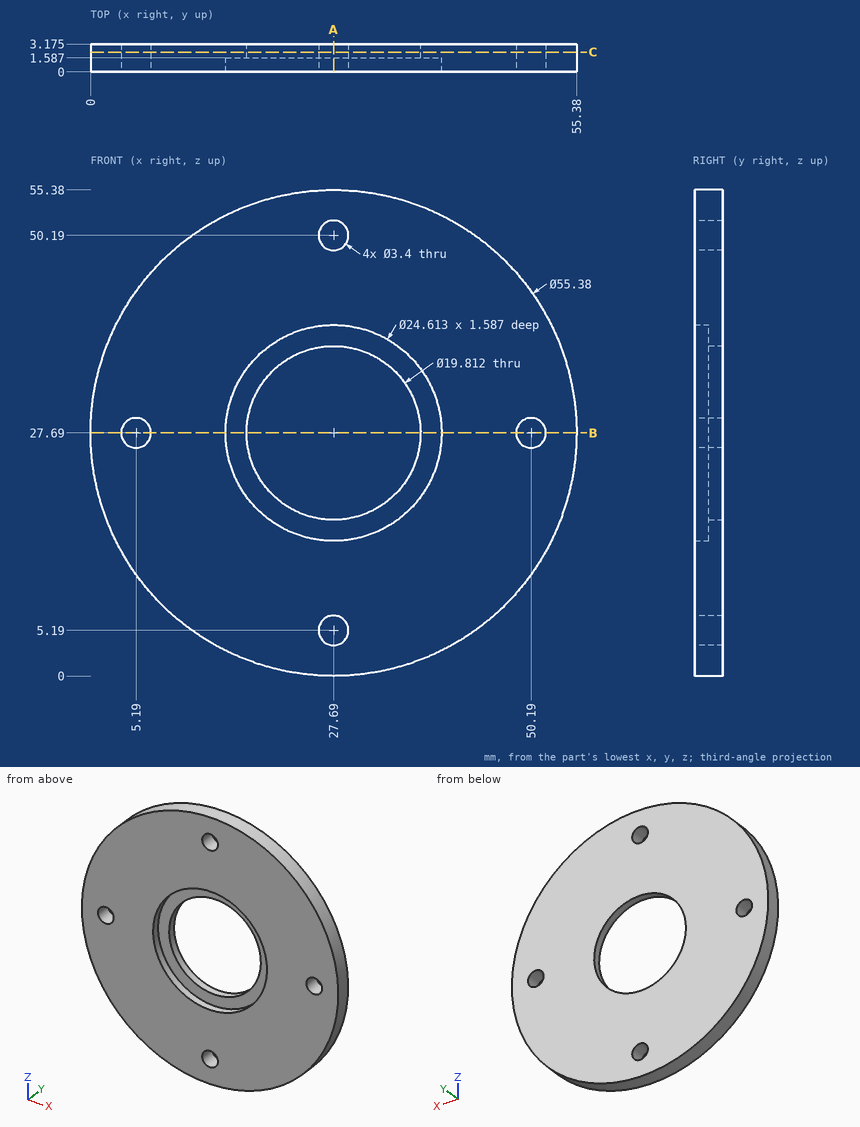
Study the drawing (mm; zero at the part's minimum x, y, z) and answer. Coordinates: 2 decimals unless noted, no trailing zeros. Loops run counter-clockwise (first coordinate to the right, second up) from the corner with the lowest first, then second, coordinate; pieces in that order, holes last. Notation, with made-up numbers: (-24.75, 14.5) -> (7.25, 14.5) arc R25 cw to (7.25, 49.5) -> close; hole circle Ø10 at (68, 65.25). An arc over 180 degrees is marked (long way). Answer in a Markdown table with one row per item. Add a question column.
1. The part is cut by section A-A, the plane x = 27.69. Write down the section's boundary in (y, z) (1 decimal).
2. A flat-ended cylindrical pin translates along its axis: P1, Ø2, axis at x = 50.19, z = 27.69, coming from the +Y side. Find the tip coordinate at first contact, or state that the pin passes through.
3. The part is cut by section C-C, the plane y = 2.25. Write down the section's boundary in (x, z) (1 decimal), then the cut area to 3 significant figures.
4. The part is cut by section B-B, the plane z = 27.69. Write down the section's boundary in (x, y) (1 decimal).
5. Consider line 1 (X direction, y = 2.6, z = 27.69) (1 decimal); line 2 (X direction, y = 1, z = 27.69); line 3 (X direction, y = 1.9, z = 4.5) (1 decimal). Determine where each line is inside the solid, lowest interval first. Write a range as [from, to].
Answer below:
| question | item | result |
|---|---|---|
| 1 | outline | (0, 0) -> (3.2, 0) -> (3.2, 3.5) -> (0, 3.5) -> close; (0, 6.9) -> (3.2, 6.9) -> (3.2, 17.8) -> (1.6, 17.8) -> (1.6, 15.4) -> (0, 15.4) -> close; (0, 40) -> (1.6, 40) -> (1.6, 37.6) -> (3.2, 37.6) -> (3.2, 48.5) -> (0, 48.5) -> close; (0, 51.9) -> (3.2, 51.9) -> (3.2, 55.4) -> (0, 55.4) -> close |
| 2 | P1 | through |
| 3 | outline | circle Ø55.4 at (27.7, 27.7); hole circle Ø3.4 at (5.2, 27.7); hole circle Ø19.8 at (27.7, 27.7); hole circle Ø3.4 at (27.7, 5.2); hole circle Ø3.4 at (27.7, 50.2); hole circle Ø3.4 at (50.2, 27.7) |
| 3 | area | 2,060 mm2 |
| 4 | outline | (0, 0) -> (3.5, 0) -> (3.5, 3.2) -> (0, 3.2) -> close; (6.9, 0) -> (15.4, 0) -> (15.4, 1.6) -> (17.8, 1.6) -> (17.8, 3.2) -> (6.9, 3.2) -> close; (37.6, 1.6) -> (40, 1.6) -> (40, 0) -> (48.5, 0) -> (48.5, 3.2) -> (37.6, 3.2) -> close; (51.9, 0) -> (55.4, 0) -> (55.4, 3.2) -> (51.9, 3.2) -> close |
| 5 | line 1 | [0, 3.5], [6.9, 17.8], [37.6, 48.5], [51.9, 55.4] |
| 5 | line 2 | [0, 3.49], [6.89, 15.38], [40, 48.49], [51.89, 55.38] |
| 5 | line 3 | [12.6, 26.1], [29.2, 42.8] |
